For this review, take the finished solid that the model builds, in its own axes (mm). Face numbers are marked on the shaded views. A direction names the side the tool comes from. Coordinates: 2 decimals unless noted, no trailing zeros. Write each loop counter-clockwise with the first axis right and the second up, starting at its lowest first coordinate (ties: lowest second). Pieces come first, ordered by that corner, then holes.
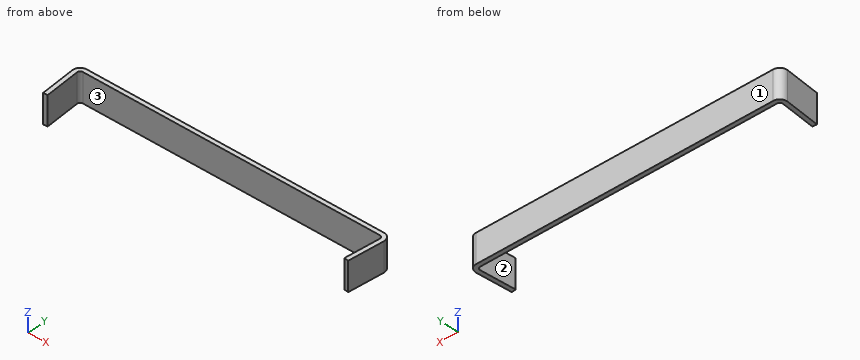
```python
from build123d import *

# Parameters (mm, degrees)
SKETCH1_W                      = 210
SKETCH1_H                      = 20
BASE_FLANGE1_DEPTH             = 3
EDGE_FLANGE1_STRIP_CUT_DEPTH   = 20
EDGE_FLANGE1_STRIP_CUT_2_DEPTH = 20
EDGE_FLANGE1_DEPTH             = 20
EDGE_FLANGE1_BEND_DEPTH        = 20


# Sheet-metal steps are written as plain solids
with BuildPart() as part:
    # Sketch1 → Base-Flange1 (new body)
    with BuildSketch(Plane(origin=(0, 0, 0), x_dir=(1, 0, 0), z_dir=(0, 1, 0))):
        Rectangle(SKETCH1_W, SKETCH1_H)
    extrude(amount=-BASE_FLANGE1_DEPTH)

    # Edge-Flange1 strip (across the edge) → Edge-Flange1 strip cut (cut)
    with BuildSketch(Plane(origin=(-105, -3, 10), x_dir=(0.9961946980917459, 0.08715574274765482, 0), z_dir=(0, 0, -1))):
        Polygon((-14.95871317, -4.320177336), (2.435778714, -2.798356488), (2.174311485, 0.190227606), (-15.220180398, -1.331593242), align=None)
    extrude(amount=EDGE_FLANGE1_STRIP_CUT_DEPTH, mode=Mode.SUBTRACT)

    # Edge-Flange1 strip 2 (across the edge) → Edge-Flange1 strip cut 2 (cut)
    with BuildSketch(Plane(origin=(105, -3, -10), x_dir=(-0.9961946980917459, 0.08715574274765482, 0), z_dir=(0, 0, 1))):
        Polygon((-14.95871317, -4.320177336), (2.435778714, -2.798356488), (2.174311485, 0.190227606), (-15.220180398, -1.331593242), align=None)
    extrude(amount=EDGE_FLANGE1_STRIP_CUT_2_DEPTH, mode=Mode.SUBTRACT)

    # Edge-Flange1 section (across the edge) → Edge-Flange1 (add)
    with BuildSketch(Plane(origin=(-105, -3, 10), x_dir=(0.9961946980917459, 0.08715574274765482, 0), z_dir=(0, 0, -1))):
        with BuildLine():
            Line((-3, 2.182617002), (-3, 26.726074497))
            Line((-3, 26.726074497), (0, 26.726074497))
            Line((0, 26.726074497), (0, 2.182617002))
            ThreePointArc((0, 2.182617002), (0.648819585, 0.708062329), (2.174311485, 0.190227606))
            Line((2.174311485, 0.190227606), (2.435778714, -2.798356488))
            ThreePointArc((2.435778714, -2.798356488), (-1.377951038, -1.503769682), (-3, 2.182617002))
        make_face()
    extrude(amount=EDGE_FLANGE1_DEPTH)

    # Edge-Flange1 section 2 (across the edge) → Edge-Flange1 bend (add)
    with BuildSketch(Plane(origin=(105, -3, -10), x_dir=(-0.9961946980917459, 0.08715574274765482, 0), z_dir=(0, 0, 1))):
        with BuildLine():
            Line((-3, 2.182617002), (-3, 26.726074497))
            Line((-3, 26.726074497), (0, 26.726074497))
            Line((0, 26.726074497), (0, 2.182617002))
            ThreePointArc((0, 2.182617002), (0.648819585, 0.708062329), (2.174311485, 0.190227606))
            Line((2.174311485, 0.190227606), (2.435778714, -2.798356488))
            ThreePointArc((2.435778714, -2.798356488), (-1.377951038, -1.503769682), (-3, 2.182617002))
        make_face()
    extrude(amount=EDGE_FLANGE1_BEND_DEPTH)


solid = part.part
```
Q1. For probe 1 along Y at (x, z) = (44, -4.5); probe 2 along X at (y, z) = (-8.5, 2.25); probe 3 along X at (y, z) = (-20.25, -1), list the stretches that pass through material, from the lowest coordinate up.
Ans:
probe 1: y = -3 to 0
probe 2: x = -107.53 to -104.52, 104.52 to 107.53
probe 3: x = -106.5 to -103.49, 103.49 to 106.5
Q2. Tool access review of the marked faces 1, 2 and 3: name each direction out of +Z, -Z, +X, -X, +Y, -Y from which nothing blocks a thin tool from reaching the whole face with its end or side.
Ans:
face 1: +Z, -Z, +X, -X, +Y
face 2: +Z, -Z
face 3: +Z, -Z, -Y
Q3. Clearance check with flat-ended pins moving along their axes: pin 1 Ø1.5 at (x, z) = (-77, 2) entering from -Y; pin 2 Ø10 at (y, z) = (-13.5, -1.5) entering from -X; pin 3 Ø8 at (y, z) = (-23.5, -4.5) entering from +X. State where each tip first meets the part, or that it passes through.
Ans:
pin 1: stops at y = -3
pin 2: stops at x = -107.53
pin 3: stops at x = 106.57
Q4. Add section A-A (z = -7). State the section outline as (x, y) points, then the cut area to 3 significant figures.
Ans:
outline: (-107.8, -5.44) - (-105.66, -29.89) - (-102.67, -29.62) - (-104.81, -5.17) arc R2 cw to (-102.82, -3) - (102.82, -3) arc R2 cw to (104.81, -5.17) - (102.67, -29.62) - (105.66, -29.89) - (107.8, -5.44) arc R5 ccw to (102.82, 0) - (-102.82, 0) arc R5 ccw to start
area: 799 mm2
Q5. Add section B-B (y = -18.5). State the section outline as (x, z) points.
Ans:
outline: (-106.66, -10) - (-103.64, -10) - (-103.64, 10) - (-106.66, 10) - close; (103.64, -10) - (106.66, -10) - (106.66, 10) - (103.64, 10) - close
Q6. Add section C-C (x = 33). State the section outline as (y, z) points, then the cut area to 3 significant figures.
Ans:
outline: (-3, -10) - (0, -10) - (0, 10) - (-3, 10) - close
area: 60.0 mm2
